Source: CAD feature listing. Evaluate the final solid. Frame: model axes, mm. A direction names the side the tool comes from. Round coordinates to 2 decimals unless told otherwise and drop trailing zeros. Write each loop counter-clockwise with the first axis right and the second up, starting at its lowest first coordinate (ties: lowest second). Pieces come first, ordered by that corner, then holes. Notation, with made-up numbers: M -13.5,-23 L 2.5,-23 A25 cw 2.5,-2 Z; hole C 32,-18 d2. An arc over 180 degrees is marked long. Use a Markdown table: item, result.
```python
from build123d import *

# Parameters (mm, degrees)
BASE_FLANGE1_DEPTH            = 4
EDGE_FLANGE1_STRIP_W          = 16.4
EDGE_FLANGE1_STRIP_H          = 4
EDGE_FLANGE1_STRIP_CUT_DEPTH  = 414.766345977
EDGE_FLANGE1_RELIEF_W         = 18.4
EDGE_FLANGE1_RELIEF_H         = 2
EDGE_FLANGE1_RELIEF_CUT_DEPTH = 4
EDGE_FLANGE1_DEPTH            = 414.766345977


# Sheet-metal steps are written as plain solids
with BuildPart() as part:
    # Sketch1 → Base-Flange1 (new body)
    with BuildSketch(Plane(origin=(0, 0, 0), x_dir=(0, 0, -1), z_dir=(1, 0, 0))):
        with BuildLine():
            Line((175.194547185, 25.010679354), (-239.571798792, 25.010679354))
            Line((-239.571798792, 25.010679354), (-251.844435082, -2.304137004))
            ThreePointArc((-251.844435082, -2.304137004), (-252.071577805, -6.636355429), (-249.318881936, -9.989320646))
            Line((-249.318881936, -9.989320646), (184.941630328, -9.989320646))
            ThreePointArc((184.941630328, -9.989320646), (187.694326197, -6.636355429), (187.467183475, -2.304137004))
            Line((187.467183475, -2.304137004), (175.194547185, 25.010679354))
        make_face()
    extrude(amount=-BASE_FLANGE1_DEPTH)

    # Edge-Flange1 strip (across the edge) → Edge-Flange1 strip cut (cut)
    with BuildSketch(Plane(origin=(-4, 25.010679354, 239.571798792), x_dir=(0, -1, 0), z_dir=(0, 0, -1))):
        with Locations((-4, -2)):
            Rectangle(EDGE_FLANGE1_STRIP_W, EDGE_FLANGE1_STRIP_H)
    extrude(amount=EDGE_FLANGE1_STRIP_CUT_DEPTH, mode=Mode.SUBTRACT)

    # Edge-Flange1 relief (on the sheet) → Edge-Flange1 relief cut (cut)
    with BuildSketch(Plane(origin=(-4, 20.810679354, 239.571798792), x_dir=(0, -1, 0), z_dir=(-1, 0, 0))):
        with Locations((-7.2, 1)):
            Rectangle(EDGE_FLANGE1_RELIEF_W, EDGE_FLANGE1_RELIEF_H)
        with Locations((-7.2, -415.766345977)):
            Rectangle(EDGE_FLANGE1_RELIEF_W, EDGE_FLANGE1_RELIEF_H)
    extrude(amount=-EDGE_FLANGE1_RELIEF_CUT_DEPTH, mode=Mode.SUBTRACT)

    # Edge-Flange1 section (across the edge) → Edge-Flange1 (add)
    with BuildSketch(Plane(origin=(-4, 25.010679354, 239.571798792), x_dir=(0, -1, 0), z_dir=(0, 0, -1))):
        with BuildLine():
            Line((0, 0.2), (0, 31))
            Line((0, 31), (4, 31))
            Line((4, 31), (4, 0.2))
            ThreePointArc((4, 0.2), (4.058578644, 0.058578644), (4.2, 0))
            Line((4.2, 0), (4.2, -4))
            ThreePointArc((4.2, -4), (1.230151519, -2.769848481), (0, 0.2))
        make_face()
    extrude(amount=EDGE_FLANGE1_DEPTH)


solid = part.part
```
Q1. Section A-A on z = -114. Return loops of the section in (x, y), plus the area to 3 significant figures.
Results are:
| item | result |
|---|---|
| outline | M -35,21.01 L -4.2,21.01 A0.2 cw -4,20.81 L -4,-9.99 L 0,-9.99 L 0,20.81 A4.2 ccw -4.2,25.01 L -35,25.01 Z |
| area | 260 mm^2 |
Q2. Line query: L1, parallel to Y at x = -12, z = 158; L2, parallel to X at y = 13, z = -124.5; L3, parallel to Y at x = -1.5, z = 29.5. Output: solid intervals per line, ascending.
Results are:
| item | result |
|---|---|
| L1 | 21.01 to 25.01 |
| L2 | -4 to 0 |
| L3 | -9.99 to 24.03 |
Q3. Section C-C on y = 3. Return loops of the section in (x, z).
Results are:
| item | result |
|---|---|
| outline | M -4,-185.08 L 0,-185.08 L 0,249.46 L -4,249.46 Z |
Q4. First-contact query: pin 1 Ø5 at (x, y) = (-8.5, 16) entering from -Z; pin 2 Ø4 at (x, z) = (-9.5, -43) entering from -Y; pin 3 Ø1.6 at (x, z) = (-1, 240.5) entering from +Y; pin 4 Ø1.9 at (x, y) = (-21.5, 21.5) entering from -Z. Flat tips, straight axial feed; report the tip coordinate or a pass-through.
Results are:
| item | result |
|---|---|
| pin 1 | through |
| pin 2 | y = 21.01 |
| pin 3 | y = 18.81 |
| pin 4 | z = -175.19 |
Q5. Reachability of faces 1 (the flat face through (-1.97, 8.97, -182.4)), 2 (the flat face through (-20, 21.011, 35)) from +Z, -Z, +X, -X, +Y, -Y: full face, straight path, thin tool, end or side. Return the list, or none.
Results are:
| item | result |
|---|---|
| face 1 | -Z, +X, -X, +Y |
| face 2 | +Z, -Z, -X, -Y |
Q6. Section B-B on x = -30. Return loops of the section in (y, z), plus the area to 3 significant figures.
Results are:
| item | result |
|---|---|
| outline | M 21.01,-175.19 L 25.01,-175.19 L 25.01,239.57 L 21.01,239.57 Z |
| area | 1,660 mm^2 |
